Verification items for the finished model (mm, model axes). A direction names the side the tool comes from. Round coordinates to 2 decimals unless told otherwise and drop trailing zeros. Loops run counter-clockwise (first coordinate to the right, second up) from the corner with the lowest first, then second, coordinate; pieces in that order, holes last. Notation, with made-up numbers: M 58,48.5 L 89,48.5 A16 cw 89,54.5 Z; hole C 60.5,55 d1. An arc over 180 degrees is marked long. One line per item, written item: value.
from build123d import *

# Parameters (mm, degrees)
F1_DEPTH = 3
F3_DEPTH = 100
F4_DEPTH = 100


with BuildPart() as f1:
    # F0 (on Top) → F1 (new body)
    with BuildSketch(Plane.XY):
        with BuildLine():
            ThreePointArc((50, 20), (47.071068, 27.071068), (40, 30))
            Line((40, 30), (-40, 30))
            ThreePointArc((-40, 30), (-47.071068, 27.071068), (-50, 20))
            Line((-50, 20), (-50, -20))
            ThreePointArc((-50, -20), (-47.071068, -27.071068), (-40, -30))
            Line((-40, -30), (40, -30))
            ThreePointArc((40, -30), (47.071068, -27.071068), (50, -20))
            Line((50, -20), (50, 20))
        make_face()
    extrude(amount=F1_DEPTH)

    # F0 (on Top) → F3 (join)
    with BuildSketch(Plane.XY):
        with BuildLine():
            ThreePointArc((50, 20), (47.071068, 27.071068), (40, 30))
            Line((40, 30), (-40, 30))
            ThreePointArc((-40, 30), (-47.071068, 27.071068), (-50, 20))
            Line((-50, 20), (-50, -20))
            ThreePointArc((-50, -20), (-47.071068, -27.071068), (-40, -30))
            Line((-40, -30), (40, -30))
            ThreePointArc((40, -30), (47.071068, -27.071068), (50, -20))
            Line((50, -20), (50, 20))
        make_face()
    extrude(amount=F3_DEPTH)

    # F2 (on face) → F4 (cut)
    with BuildSketch(Plane.XY.offset(3)):
        with BuildLine():
            Line((-47, 20), (-47, -20))
            ThreePointArc((-47, -20), (-44.949747, -24.949747), (-40, -27))
            Line((-40, -27), (40, -27))
            ThreePointArc((40, -27), (44.949747, -24.949747), (47, -20))
            Line((47, -20), (47, 20))
            ThreePointArc((47, 20), (44.949747, 24.949747), (40, 27))
            Line((40, 27), (-40, 27))
            ThreePointArc((-40, 27), (-44.949747, 24.949747), (-47, 20))
        make_face()
    extrude(amount=F4_DEPTH, mode=Mode.SUBTRACT)


solid = f1.part
(1) Thickness scan on L1, parallel to X at y = -12, z = 23; L2, parallel to Y at x = -19, z = 56; L3, parallel to Z at x = -29, y = 25. Record the ranges inside material, lowest first. Write a range as from..to.
Completed:
L1: x = -50..-47, 47..50
L2: y = -30..-27, 27..30
L3: z = 0..3
(2) Tool access check on faces 1 (the face through (46.99, -27.15, 49.3)), 2 (the face through (-44.9, 25, 50.8)). Record the directions out of +Z, -Z, +X, -X, +Y, -Y that give a thin tool (end or side, any length) a straight path to the whole face; none if there is none.
Completed:
face 1: +Z, -Z, +X, -Y
face 2: +Z
(3) Mould release check, pull along X, two halves, no side actions. Record for faces 3 (the face through (-1, -30, 49)), 4 (the face through (-47.15, -26.99, 49.3)), 5 (the face through (-1, -27, 51)): +X half, -X half, draft (parallel to the pull), parting line (faces both ways), or undercut.
Completed:
face 3: draft
face 4: -X half
face 5: undercut
(4) Sectioned sample at B-B on x = -26. Enter the section's corners in (y, z).
Completed:
outline: M -30,0 L 30,0 L 30,100 L 27,100 L 27,3 L -27,3 L -27,100 L -30,100 Z
(5) Depth check by flat-ended pin: pin 1 Ø16 at (x, y) = (-19, -6) entering from +Z. Enter the tip coordinate at first touch or a pass-through.
Completed:
pin 1: stops at z = 3
(6) Sectioned sample at C-C on y = 1.5. Enter the section's corners in (x, z).
Completed:
outline: M -50,0 L 50,0 L 50,100 L 47,100 L 47,3 L -47,3 L -47,100 L -50,100 Z
(7) Sectioned sample at A-A on z = 65. Enter the section's corners in (x, y).
Completed:
outline: M -50,-20 A10 ccw -40,-30 L 40,-30 A10 ccw 50,-20 L 50,20 A10 ccw 40,30 L -40,30 A10 ccw -50,20 Z; hole M -47,-20 A7 ccw -40,-27 L 40,-27 A7 ccw 47,-20 L 47,20 A7 ccw 40,27 L -40,27 A7 ccw -47,20 Z
